```python
from build123d import *

# Parameters (mm, degrees)
SKETCH_1_R                      = 8
EXTRUDE_1_DEPTH                 = 4
SKETCH_7_R                      = 3.333333333
CUT_EXTRUDE_3_DEPTH             = 33.771939216
SKETCH_8_R                      = 2
CUT_EXTRUDE_4_DEPTH             = 33.771939216
EXTRUDE_START                   = 28
SKETCH_9_R                      = 3
SKETCH_9_R_2                    = 2
EXTRUDE_2_DEPTH                 = 4
EXTRUDE_3_REACH                 = 47.629
SKETCH_10_W                     = 13.024468831
SKETCH_10_H                     = 3.5
SKETCH_11_W                     = 28
SKETCH_11_H                     = 3.5
EXTRUDE_4_DEPTH                 = 15
SCALE_1_SCALE                   = 1.5
CUT_EXTRUDE_5_DEPTH             = 42
SKETCH_17_R                     = 6
CUT_EXTRUDE_6_DEPTH             = 1.4
SKETCH_18_R                     = 5
CUT_EXTRUDE_7_DEPTH             = 5
CUT_EXTRUDE_8_REACH             = 72.05
SKETCH_19_R                     = 2
CUT_EXTRUDE_8_DIRECTION_2_DEPTH = 71.050046232
FILLET_1_R                      = 5
SKETCH_21_R                     = 3.5
CUT_EXTRUDE_9_DEPTH             = 3


with BuildPart() as part:
    # Sketch 1 → Extrude 1 (new body)
    with BuildSketch(Plane(origin=(0, 0, 0), x_dir=(0, 0, -1), z_dir=(1, 0, 0))):
        with BuildLine():
            ThreePointArc((-7, -15), (-9.343145751, -20.656854249), (-15, -23))
            Line((-15, -23), (14.121578143, -23))
            Line((14.121578143, -23), (14.121578143, -19.5))
            Line((14.121578143, -19.5), (1.097109312, -19.5))
            ThreePointArc((1.097109312, -19.5), (1.721982831, -12.038332525), (5.650082252, -5.66361815))
            ThreePointArc((5.650082252, -5.66361815), (-4.947792662, -6.286441583), (-6.832692698, 4.161046803))
            ThreePointArc((-6.832692698, 4.161046803), (-12.258618637, -2.741381363), (-19.161046803, -8.167307302))
            ThreePointArc((-19.161046803, -8.167307302), (-11.081350642, -8.025461506), (-7, -15))
        make_face()
        with Locations((-15, -15)):
            Circle(SKETCH_1_R)
        Circle(SKETCH_1_R)
    extrude(amount=EXTRUDE_1_DEPTH)

    # Sketch 7 → Cut-Extrude 3 (cut, through all)
    with BuildSketch(Plane(origin=(4, 0, 0), x_dir=(0, 0, -1), z_dir=(1, 0, 0))):
        Circle(SKETCH_7_R)
    extrude(amount=-CUT_EXTRUDE_3_DEPTH, mode=Mode.SUBTRACT)

    # Sketch 8 → Cut-Extrude 4 (cut, through all)
    with BuildSketch(Plane(origin=(4, 0, 0), x_dir=(0, 0, -1), z_dir=(1, 0, 0))):
        with Locations((-15, -15)):
            Circle(SKETCH_8_R)
    extrude(amount=-CUT_EXTRUDE_4_DEPTH, mode=Mode.SUBTRACT)


with BuildPart() as body_2:
    # Sketch 9 → Extrude 2 (new body)
    with BuildSketch(Plane.ZY.offset(EXTRUDE_START)):
        with BuildLine():
            Line((-1.097109312, -19.5), (-14.121578143, -19.5))
            Line((-14.121578143, -19.5), (-14.121578143, -23))
            Line((-14.121578143, -23), (15, -23))
            ThreePointArc((15, -23), (22.702646999, -17.160839931), (19.161046803, -8.167307302))
            ThreePointArc((19.161046803, -8.167307302), (12.258618637, -2.741381363), (6.832692698, 4.161046803))
            ThreePointArc((6.832692698, 4.161046803), (-4.947792662, 6.286441583), (-5.650082252, -5.66361815))
            ThreePointArc((-5.650082252, -5.66361815), (-1.721982831, -12.038332525), (-1.097109312, -19.5))
        make_face()
        Circle(SKETCH_9_R, mode=Mode.SUBTRACT)
        with Locations(Location((15, -15, 0), (0, 0, 180))):
            Circle(SKETCH_9_R_2, mode=Mode.SUBTRACT)
    extrude(amount=EXTRUDE_2_DEPTH)

    # Sketch 10 → Extrude 3 (add, up to next)
    with BuildSketch(Plane.ZY, mode=Mode.PRIVATE) as extrude_3_sk1:
        with Locations((-7.609343728, -21.25)):
            Rectangle(SKETCH_10_W, SKETCH_10_H)
    extrude_3_tool1 = extrude(extrude_3_sk1.sketch, amount=EXTRUDE_3_REACH, mode=Mode.PRIVATE) - body_2.part

    add(part.part)  # Extrude 3 merges part
    add(extrude_3_tool1.solids().sort_by_distance((0, -21.25, -7.609344))[0])

    # Sketch 11 → Extrude 4 (add)
    with BuildSketch(Plane.XY.offset(-1.097109312)):
        with Locations((-14, -21.25)):
            Rectangle(SKETCH_11_W, SKETCH_11_H)
    extrude(amount=EXTRUDE_4_DEPTH)


with BuildPart() as body_2_1:
    # Scale 1: scaled about (-14.05550312, -14.324036163, 3.699652839)
    add(body_2.part.scale(SCALE_1_SCALE).moved(Location((7.02775156, 7.162018082, -1.84982642))))

    # Sketch 13 → Cut-Extrude 5 (cut)
    with BuildSketch(Plane(origin=(-34.97224844, 0, 0), x_dir=(0, 0, -1), z_dir=(1, 0, 0))):
        with BuildLine():
            Line((-14.697233131, -22.087981919), (-19.004509613, -22.087981919))
            Line((-19.004509613, -22.087981919), (-19.004509613, -24.186246726))
            ThreePointArc((-19.004509613, -24.186246726), (-16.708679438, -23.42900311), (-14.697233131, -22.087981919))
        make_face()
    extrude(amount=CUT_EXTRUDE_5_DEPTH, mode=Mode.SUBTRACT)

    # Sketch 17 → Cut-Extrude 6 (cut)
    with BuildSketch(Plane.ZY.offset(40.97224844)):
        with Locations((20.650173581, -15.337981919)):
            Circle(SKETCH_17_R)
    extrude(amount=-CUT_EXTRUDE_6_DEPTH, mode=Mode.SUBTRACT)

    # Sketch 18 → Cut-Extrude 7 (cut)
    with BuildSketch(Plane(origin=(13.02775156, 0, 0), x_dir=(0, 0, -1), z_dir=(1, 0, 0))):
        with Locations((-20.650173581, -15.337981919)):
            Circle(SKETCH_18_R)
    extrude(amount=-CUT_EXTRUDE_7_DEPTH, mode=Mode.SUBTRACT)

    # Sketch 19 → Cut-Extrude 8 (cut, up to next)
    with BuildSketch(Plane.XZ.offset(27.337981919), mode=Mode.PRIVATE) as cut_extrude_8_sk1:
        with Locations(Location((-0.97224844, -12.01384201, 0), (0, 0, 90))):
            Circle(SKETCH_19_R)
    cut_extrude_8_tool1 = extrude(cut_extrude_8_sk1.sketch, amount=-CUT_EXTRUDE_8_REACH, mode=Mode.PRIVATE) & body_2_1.part
    # Sketch 19 → Cut-Extrude 8 (cut, up to next)
    with BuildSketch(Plane.XZ.offset(27.337981919), mode=Mode.PRIVATE) as cut_extrude_8_sk2:
        with Locations(Location((-26.97224844, -12.01384201, 0), (0, 0, 90))):
            Circle(SKETCH_19_R)
    cut_extrude_8_tool2 = extrude(cut_extrude_8_sk2.sketch, amount=-CUT_EXTRUDE_8_REACH, mode=Mode.PRIVATE) & body_2_1.part
    # Sketch 19 → Cut-Extrude 8 (cut, up to next)
    with BuildSketch(Plane.XZ.offset(27.337981919), mode=Mode.PRIVATE) as cut_extrude_8_sk3:
        with Locations(Location((-26.97224844, 7.98615799, 0), (0, 0, 90))):
            Circle(SKETCH_19_R)
    cut_extrude_8_tool3 = extrude(cut_extrude_8_sk3.sketch, amount=-CUT_EXTRUDE_8_REACH, mode=Mode.PRIVATE) & body_2_1.part
    # Sketch 19 → Cut-Extrude 8 (cut, up to next)
    with BuildSketch(Plane.XZ.offset(27.337981919), mode=Mode.PRIVATE) as cut_extrude_8_sk4:
        with Locations(Location((-0.97224844, 7.98615799, 0), (0, 0, 90))):
            Circle(SKETCH_19_R)
    cut_extrude_8_tool4 = extrude(cut_extrude_8_sk4.sketch, amount=-CUT_EXTRUDE_8_REACH, mode=Mode.PRIVATE) & body_2_1.part
    add(cut_extrude_8_tool1.solids().sort_by_distance((-0.972248, -27.337982, -12.013842))[0], mode=Mode.SUBTRACT)
    add(cut_extrude_8_tool2.solids().sort_by_distance((-26.972248, -27.337982, -12.013842))[0], mode=Mode.SUBTRACT)
    add(cut_extrude_8_tool3.solids().sort_by_distance((-26.972248, -27.337982, 7.986158))[0], mode=Mode.SUBTRACT)
    add(cut_extrude_8_tool4.solids().sort_by_distance((-0.972248, -27.337982, 7.986158))[0], mode=Mode.SUBTRACT)

    # Sketch 19 → Cut-Extrude 8 direction 2 (cut)
    with BuildSketch(Plane.XZ.offset(27.337981919)):
        with Locations(Location((-0.97224844, -12.01384201, 0), (0, 0, 90))):
            Circle(SKETCH_19_R)
        with Locations(Location((-26.97224844, -12.01384201, 0), (0, 0, 90))):
            Circle(SKETCH_19_R)
        with Locations(Location((-26.97224844, 7.98615799, 0), (0, 0, 90))):
            Circle(SKETCH_19_R)
        with Locations(Location((-0.97224844, 7.98615799, 0), (0, 0, 90))):
            Circle(SKETCH_19_R)
    extrude(amount=CUT_EXTRUDE_8_DIRECTION_2_DEPTH, mode=Mode.SUBTRACT)

    # Fillet 1
    fillet_1_edges = [body_2_1.edges().sort_by_distance(p)[0] for p in [
        (13.02775156, -24.712981919, -23.032193634),
        (-40.97224844, -24.712981919, -23.032193634),
    ]]
    fillet(fillet_1_edges, radius=FILLET_1_R)

    # Sketch 21 → Cut-Extrude 9 (cut)
    with BuildSketch(Plane(origin=(0, -22.087981919, 0), x_dir=(1, 0, 0), z_dir=(0, 1, 0))):
        with Locations(Location((-26.97224844, 12.01384201, 0), (0, 0, 270))):
            Circle(SKETCH_21_R)
        with Locations(Location((-0.97224844, 12.01384201, 0), (0, 0, 270))):
            Circle(SKETCH_21_R)
        with Locations(Location((-0.97224844, -7.98615799, 0), (0, 0, 270))):
            Circle(SKETCH_21_R)
        with Locations(Location((-26.97224844, -7.98615799, 0), (0, 0, 270))):
            Circle(SKETCH_21_R)
    extrude(amount=-CUT_EXTRUDE_9_DEPTH, mode=Mode.SUBTRACT)


solid = body_2_1.part
```
Build history of the part. All positions in model axes, mm. A direction names the side the tool comes from. Give positions to 0.01 mm unless a question says otherwise; leave off trailing zeros. Order: outer loops, then holes, each group sorted by start corner. A loop starts at its lowest first (then second) coordinate and runs counter-clockwise, first axis right, second up. Notation, with made-up numbers: M 39,2 L 50,2 A16 cw 50,16 Z; hole C -38.5,-15.5 d6. An arc over 180 degrees is marked long. Return JSON: item names as keys, results as strings.
Q1. 3-axis set-ups, long thin cutter, end or side, ignore diameter. For faces 1 (the face through (-37.9, 16.8, -9)), 2 (the face through (10.1, 11.4, -4.5)), 3 (the face through (0.079, -23.567, 11.325)): which of +Z, -Z, +X, -X, +Y, -Y reach the whole face in a straight line?
Answer list:
{"face 1": "+X, -X", "face 2": "+X", "face 3": "+Y"}
Q2. Wall check: probe 1 along X at (y, z) = (-23, 29.5); probe 2 along X at (y, z) = (-18, 16.5); probe 3 along Y at (x, z) = (5.5, -17.5). Give the ranges that are in metal, low to high. Write a range as from..to.
Answer list:
{"probe 1": "x = -40.97..-34.97, 7.03..13.03", "probe 2": "x = -39.57..-34.97, 7.03..8.03", "probe 3": "y = -27.34..-22.09"}
Q3. Two-plate mould, pull along Y, no slides. Class faces 4 (the face through (-39.572, -18, 23)), 5 (the face through (7.028, -4, 10)), 6 (the face through (-28.5, -25.088, 9.5)): pulls with the +Y half, pulls with the -Y half, needs draft (parallel to the pull), parting line crosses it, or undercut.
Answer list:
{"face 4": "undercut", "face 5": "needs draft", "face 6": "pulls with the +Y half"}
Q4. Band-saw the part on D-D (z = -4.5). Give the cut face in (x, y).
Answer list:
{"outline": "M -40.97,-27.34 L 13.03,-27.34 L 13.03,-22.09 L -40.97,-22.09 Z; M -40.97,-10.69 L -34.97,-10.69 L -34.97,3.53 L -40.97,3.53 Z; M -40.97,10.8 L -34.97,10.8 L -34.97,18.87 L -40.97,18.87 Z; M 7.03,-10.69 L 13.03,-10.69 L 13.03,2.92 L 7.03,2.92 Z; M 7.03,11.4 L 13.03,11.4 L 13.03,18.87 L 7.03,18.87 Z"}
Q5. Band-saw the part on B-B (y = 1). Give the cut face in (x, z), then the cut area to 3 significant figures.
Answer list:
{"outline": "M -40.97,-12.15 L -34.97,-12.15 L -34.97,18.7 L -40.97,18.7 Z; M 7.03,-12.15 L 13.03,-12.15 L 13.03,18.7 L 7.03,18.7 Z", "area": "370 mm^2"}
Q6. Band-saw the part on C-C (y = 8). Give the cut face in (x, z), then the cut area to 3 significant figures.
Answer list:
{"outline": "M -40.97,-13.82 L -34.97,-13.82 L -34.97,-6.27 L -40.97,-6.27 Z; M -40.97,2.57 L -34.97,2.57 L -34.97,12.15 L -40.97,12.15 Z; M 7.03,-13.82 L 13.03,-13.82 L 13.03,-6.78 L 7.03,-6.78 Z; M 7.03,3.08 L 13.03,3.08 L 13.03,12.15 L 7.03,12.15 Z", "area": "199 mm^2"}
Q7. Band-saw the part on A-A (z = 22). Give the cut face in (x, y), then the cut area to 3 significant figures.
Answer list:
{"outline": "M -40.97,-27.26 L -34.97,-27.26 L -34.97,-18.02 L -39.57,-18.02 L -39.57,-21.18 L -40.97,-21.18 Z; M -40.97,-9.49 L -39.57,-9.49 L -39.57,-12.66 L -34.97,-12.66 L -34.97,-1.74 L -40.97,-1.74 Z; M 7.03,-27.26 L 13.03,-27.26 L 13.03,-20.15 L 8.03,-20.15 L 8.03,-18.02 L 7.03,-18.02 Z; M 7.03,-12.66 L 8.03,-12.66 L 8.03,-10.52 L 13.03,-10.52 L 13.03,-1.74 L 7.03,-1.74 Z", "area": "212 mm^2"}
Q8. Flat gauge pins, fed straight in: pin 1 (3.5 mm diameter, centred on x = -27.5, z = 7.5, fed in from +Y); pin 2 (5.5 mm diameter, centred on x = -28.5, z = -11.5, fed in from +Y); pin 3 (12 mm diameter, centred on x = -25, y = 14, fed in from -Z); pin 4 (9.5 mm diameter, centred on y = -15.34, z = 20.65, fed in from -X). Where does each tip first touch, or does it go through?
Answer list:
{"pin 1": "stops at y = -25.09", "pin 2": "stops at y = -22.09", "pin 3": "passes through", "pin 4": "stops at x = -39.57"}
